Geometry check sheet. Reference: the model listing, model coordinates, mm. A direction names the side the tool comes from. Coordinates: 2 decimals unless noted, no trailing zeros. Write each loop counter-clockwise with the first axis right and the second up, starting at its lowest first coordinate (ties: lowest second). Pieces come first, ordered by that corner, then holes. Notation, with made-up numbers: M 31.25,87.5 L 46.25,87.5 A14 ccw 46.25,92.5 Z; hole C 29.25,46.25 d11. An arc over 180 degrees is marked long. Put each result on its own line as item: value. Start each with the question number.
1) Scan lines: line 1 along X through (y, z) = (18.75, 0); line 2 along X through (y, z) = (13.5, 0); line 3 along Z through (x, y) = (-18.95, 18.95). Record each from-to range of solid material in increasing order.
2) Cross-section at B-B on x = 0. Record the cut outline in (y, z).
3) Set-up check for faces 1 (the flat face through (-0.1, 4, 17.5)), 2 (the flat face through (-9.432, 12, 12)), 3 (the flat face through (0, 4, 14)), 4 (the flat face through (0, 0, 0)), 5 (the flat face through (0, 15.661, 19)): record each of +Z, -Z, +X, -X, +Y, -Y from which the full face is reachable in a straight line by a thin tool's end or side.
4) Cross-section at D-D on z = -6. Record the cut outline in (x, y), plus the area to 3 significant figures.
5) Gauge pin test, flat ends, axial feed: pin 1 (8 mm diameter, centred on x = 17, y = 7.5, fed in from -Z); pin 2 (0.8 mm diameter, centred on y = 18, z = 18.5, fed in from -X); pin 3 (1.8 mm diameter, centred on x = -7, z = 12, fed in from +Y). Record the tip position at first contact, or that the pin passes through.
6) Cross-section at A-A on y = 8.25. Record the cut outline in (x, z), plus the area to 3 significant figures.
7) Cross-section at C-C on x = 18.95. Record the cut outline in (y, z), plus the area to 3 significant figures.
8) Mould release check, pull along Z, two halves, no side actions. Record for faces 6 (the flat face through (8, 4, 13)), 7 (the flat face through (-21.3, 17, 0.7)), 8 (the cylindrical face through (16.754, 18.521, -0.488)), 9 (the flat face through (0, 10, 19.401)): released by +Z, released by -Z, zero draft, split by the parting line, or undercut.
from build123d import *

# Parameters (mm, degrees)
SKETCH1_R           = 17
BOSS_EXTRUDE1_DEPTH = 20
SHELL1_T            = -2.4
SKETCH2_R           = 3.45
BOSS_EXTRUDE3_DEPTH = 3
SKETCH4_R           = 2.25
CUT_EXTRUDE1_DEPTH  = 3
SKETCH5_W           = 17.5
SKETCH5_H           = 7.7
BOSS_EXTRUDE4_DEPTH = 16
SKETCH6_W           = 16
SKETCH6_H           = 8.6
CUT_EXTRUDE2_DEPTH  = 14
SKETCH7_W           = 8.6
SKETCH7_H           = 5.8
CUT_EXTRUDE3_DEPTH  = 5
FILLET4_R           = 1
SKETCH8_W           = 18.8
SKETCH8_H           = 3
CUT_EXTRUDE4_DEPTH  = 16


with BuildPart() as part:
    # Sketch1 → Boss-Extrude1 (new body)
    with BuildSketch(Plane(origin=(0, 0, 0), x_dir=(1, 0, 0), z_dir=(0, 1, 0))):
        with Locations(Location((0, 0, 0), (0, 0, 270))):
            Circle(SKETCH1_R)
    extrude(amount=BOSS_EXTRUDE1_DEPTH)

    # Shell1
    shell1_openings = [part.faces().sort_by_distance(p)[0] for p in [
        (0, 20, 0),
    ]]
    offset(amount=SHELL1_T, openings=shell1_openings, kind=Kind.INTERSECTION)

    # Sketch2 → Boss-Extrude3 (add)
    with BuildSketch(Plane(origin=(0, 20, 0), x_dir=(1, 0, 0), z_dir=(0, 1, 0))):
        with Locations((18.659372003, 0)):
            Circle(SKETCH2_R)
        with Locations((-18.659372003, 0)):
            Circle(SKETCH2_R)
    extrude(amount=-BOSS_EXTRUDE3_DEPTH)

    # Sketch4 → Cut-Extrude1 (cut)
    with BuildSketch(Plane(origin=(0, 20, 0), x_dir=(1, 0, 0), z_dir=(0, 1, 0))):
        with Locations(Location((18.95, 0, 0), (0, 0, 270))):
            Circle(SKETCH4_R)
        with Locations(Location((-18.95, 0, 0), (0, 0, 331.816850826))):
            Circle(SKETCH4_R)
    extrude(amount=-CUT_EXTRUDE1_DEPTH, mode=Mode.SUBTRACT)

    # Sketch5 → Boss-Extrude4 (add)
    with BuildSketch(Plane(origin=(0, 20, 0), x_dir=(1, 0, 0), z_dir=(0, 1, 0))):
        with Locations((0.01757968, -15.550633972)):
            Rectangle(SKETCH5_W, SKETCH5_H)
    extrude(amount=-BOSS_EXTRUDE4_DEPTH)

    # Sketch6 → Cut-Extrude2 (cut)
    with BuildSketch(Plane(origin=(0, 20, 0), x_dir=(1, 0, 0), z_dir=(0, 1, 0))):
        with Locations((0.025977535, -14.047647825)):
            Rectangle(SKETCH6_W, SKETCH6_H)
    extrude(amount=-CUT_EXTRUDE2_DEPTH, mode=Mode.SUBTRACT)

    # Sketch7 → Cut-Extrude3 (cut)
    with BuildSketch(Plane.XY.offset(19.400633972)):
        with Locations((-0.172487463, 18.560997168)):
            Rectangle(SKETCH7_W, SKETCH7_H)
    extrude(amount=-CUT_EXTRUDE3_DEPTH, mode=Mode.SUBTRACT)

    # Fillet4
    fillet4_edges = [part.edges().sort_by_distance(p)[0] for p in [
        (0, 4, 11.700633972),
    ]]
    fillet(fillet4_edges, radius=FILLET4_R)

    # Sketch8 → Cut-Extrude4 (cut)
    with BuildSketch(Plane(origin=(0, 20, 0), x_dir=(1, 0, 0), z_dir=(0, 1, 0))):
        with Locations((-0.031709419, -11.955798022)):
            Rectangle(SKETCH8_W, SKETCH8_H)
    extrude(amount=-CUT_EXTRUDE4_DEPTH, mode=Mode.SUBTRACT)


solid = part.part
Answer key:
1. line 1: x = -22.11 to -21.2, -16.7 to -14.6, 14.6 to 16.7, 21.2 to 22.11
1. line 2: x = -17 to -14.6, 14.6 to 17
1. line 3: z = -3.44 to -2.25, 2.25 to 3.44
2. outline: M 0,-17 L 20,-17 L 20,-14.6 L 2.4,-14.6 L 2.4,14.6 L 4,14.6 L 4,13.46 L 6,13.46 L 6,18.35 L 15.66,18.35 L 15.66,19.4 L 4,19.4 L 4,17 L 0,17 Z
3. face 1: +Z, -Y
3. face 2: +Y
3. face 3: none
3. face 4: +Z, -Z, +X, -X, -Y
3. face 5: +Z, +Y
4. outline: M -15.91,0 L 15.91,0 L 15.91,20 L 13.31,20 L 13.31,2.4 L -13.31,2.4 L -13.31,20 L -15.91,20 Z
4. area: 168 mm²
5. pin 1: stops at z = -10.95
5. pin 2: stops at x = -8.73
5. pin 3: stops at y = 4
6. outline: M -8.73,14.59 A17 ccw long 8.77,14.56 L 8.77,19.4 L -8.73,19.4 Z; hole M -9.43,11.14 A14.6 ccw long 9.37,11.2 L 9.37,13.46 L 8.03,13.46 L 8.03,18.35 L -7.97,18.35 L -7.97,13.46 L -9.43,13.46 Z
6. area: 217 mm²
7. outline: M 17,-3.44 L 20,-3.44 L 20,-2.25 L 17,-2.25 Z; M 17,2.25 L 20,2.25 L 20,3.44 L 17,3.44 Z
7. area: 7.13 mm²
8. face 6: undercut
8. face 7: zero draft
8. face 8: undercut
8. face 9: released by +Z
